Source: CAD feature listing. Evaluate the final solid. Frame: model axes, mm. Coordinates: 2 decimals unless noted, no trailing zeros. Write each loop counter-clockwise with the first axis right and the second up, starting at its lowest first coordinate (ties: lowest second). Pieces come first, ordered by that corner, then holes. Notation, with made-up numbers: (-32.5, 83.5) -> (-3.5, 83.5) arc R23 ccw to (-3.5, 113.5) -> close; hole circle Ø1 at (-31, 21.5). An arc over 180 degrees is marked (long way). Write item = value, one per line.
Autodesk Inventor part; units mm, degrees
ref_plane "YZ Plane" through (0, 0, 0) normal (1, 0, 0) x (0, 1, 0)
ref_plane "XZ Plane" through (0, 0, 0) normal (0, 1, 0) x (-1, 0, 0)
ref_plane "XY Plane" through (0, 0, 0) normal (0, 0, 1) x (1, 0, 0)
sketch "Sketch1" plane through (0, 0, 0) normal (0, 1, 0) x (-1, 0, 0)
  circle A0 centre (0, 0) radius 88.9
  line L0 (0, 0) -> (121.8821, 50.4852)
  line L1 (0, 0) -> (0, 134.8176)
  line L2 (82.1329, 34.0206) -> (82.1329, -34.0206)
  line L3 (82.1329, -34.0206) -> (34.0206, -82.1329)
  line L4 (34.0206, -82.1329) -> (-34.0206, -82.1329)
  line L5 (-34.0206, -82.1329) -> (-82.1329, -34.0206)
  line L6 (-82.1329, -34.0206) -> (-82.1329, 34.0206)
  line L7 (-82.1329, 34.0206) -> (-34.0206, 82.1329)
  line L8 (-34.0206, 82.1329) -> (34.0206, 82.1329)
  line L9 (34.0206, 82.1329) -> (82.1329, 34.0206)
  dimension "d0" = 177.8
  dimension "d1" = 67.5
  dimension "d2" = 164.2658
extrude "Extrusion1" add sketch "Sketch1" along normal blind 1.5875 contours L2 L3 L4 L5 L6 L7 L8 L1 L0 | L0 L1 L8 L9
sketch "Sketch2" plane through (0, 1.5875, 0) normal (0, 1, 0) x (1, 0, 0)
  line L0 (28.575, -33.655) -> (-28.575, -33.655)
  line L1 (-28.575, -33.655) -> (-28.575, 33.655)
  line L2 (-28.575, 33.655) -> (28.575, 33.655)
  line L3 (28.575, 33.655) -> (28.575, -33.655)
  line L4 (28.575, -33.655) -> (-28.575, 33.655) construction
  line L5 (-28.575, -33.655) -> (28.575, 33.655) construction
  point P0 (0, 0)
  dimension "d5" = 57.15
  dimension "d6" = 67.31
extrude "Extrusion2" cut sketch "Sketch2" against normal through all
sketch "Sketch3" plane through (0, 1.5875, 0) normal (0, 1, 0) x (1, 0, 0)
  circle A0 centre (-69.4329, -34.0206) radius 3.6195
  line L0 (-82.1329, 34.0206) -> (-82.1329, -34.0206)
  line L1 (-91.914, 0) -> (-48.5333, 0)
  circle A1 centre (-69.4329, 34.0206) radius 3.6195
  circle A2 centre (-34.0206, -69.4329) radius 3.6195
  circle A3 centre (34.0206, -69.4329) radius 3.6195
  circle A4 centre (69.4329, -34.0206) radius 3.6195
  circle A5 centre (69.4329, 34.0206) radius 3.6195
  circle A6 centre (34.0206, 69.4329) radius 3.6195
  circle A7 centre (-34.0206, 69.4329) radius 3.6195
  point P0 (0, 0)
  dimension "d9" = 7.239
  dimension "d10" = 12.7
  dimension "d11" = 0
  dimension "d14" = 360
extrude "Extrusion3" cut sketch "Sketch3" against normal through all
properties part number "Layer"
1) Cut plane A-A, the plane z = -28. Output: boundary loops of the cut face in (x, y) (1 decimal), and give its area (3 significant figures).
Answer block:
outline = (-82.1, 0) -> (-28.6, 0) -> (-28.6, 1.6) -> (-82.1, 1.6) -> close; (28.6, 0) -> (82.1, 0) -> (82.1, 1.6) -> (28.6, 1.6) -> close
area = 170 mm2
2) First-contact query: pin 1 Ø4.5 at (x, z) = (-69.43, 34.02) entering from -Y. Flat tip, straight axial feed; report the tip coordinate or a pass-through.
Answer block:
pin_1 = through
3) Material intervals for probe 1 along X at (y, z) = (0.5, -22) (3 decimals); probe 2 along Z at (x, y) = (2, 0.5) (3 decimals); probe 3 along Z at (x, y) = (-68.5, 1), sorted ascending. Write a range as [from, to].
Answer block:
probe_1 = [-82.133, -28.575], [28.575, 82.133]
probe_2 = [-82.133, -33.655], [33.655, 82.133]
probe_3 = [-47.65, -37.52], [-30.52, 30.52], [37.52, 47.65]
4) Cut plane C-C, the plane y = 1.15. Give the number of separate pieces and of enclosed holes in the cut face, and give its area (3 significant figures).
Answer block:
separate_pieces = 1
enclosed_holes = 9
area = 18,200 mm2
5) Cut plane B-B, the plane x = -12. Output: boundary loops of the cut face in (y, z) (1 decimal), and give its area (3 significant figures).
Answer block:
outline = (0, -82.1) -> (1.6, -82.1) -> (1.6, -33.7) -> (0, -33.7) -> close; (0, 33.7) -> (1.6, 33.7) -> (1.6, 82.1) -> (0, 82.1) -> close
area = 154 mm2
6) Pull-direction query (X, two-part tool) for faces 1 (the flat face through (-58.414, 0.783, -57.74)), 2 (the cylindrical face through (72.776, 0.805, 35.407)), 3 (the flat face through (38, 0, 1)), 4 (the flat face through (57.74, 0.783, -58.414)); classes: +X half, -X half, draft (parallel to the pull), parting line (faces both ways), or undercut.
Answer block:
face_1 = -X half
face_2 = undercut
face_3 = draft
face_4 = +X half
7) Cut plane D-D, the plane x = 69. Output: boundary loops of the cut face in (y, z).
Answer block:
outline = (0, -47.15) -> (1.59, -47.15) -> (1.59, -37.61) -> (0, -37.61) -> close; (0, -30.43) -> (1.59, -30.43) -> (1.59, 30.43) -> (0, 30.43) -> close; (0, 37.61) -> (1.59, 37.61) -> (1.59, 47.15) -> (0, 47.15) -> close
